Verification items for the finished model (mm, model axes). Round coordinates to 2 decimals unless told otherwise and drop trailing zeros. Order: outer loops, then holes, each group sorted by start corner. A loop starts at its lowest first (then second) coordinate and runs counter-clockwise, first axis right, second up. Notation, with made-up numbers: M 28,1 L 65,1 A20 ccw 65,35 Z; hole C 36,70 d5. An arc over 180 degrees is marked long. One line per item, written item: value. Start each with the question number.
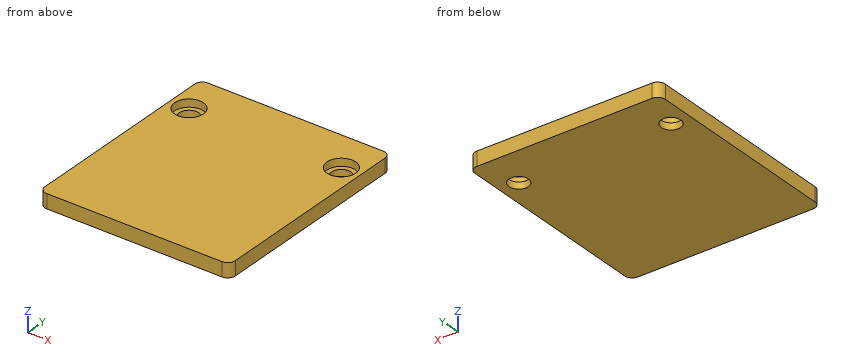
from build123d import *

# Parameters (mm, degrees)
SKETCH1_W                                        = 63.5
SKETCH1_H                                        = 71.4375
BOSS_EXTRUDE1_DEPTH                              = 4.7625
CBORE_FOR_1_4_SOCKET_HEAD_CAP_SCREW1_D           = 6.5278
CBORE_FOR_1_4_SOCKET_HEAD_CAP_SCREW1_CBORE_D     = 9.652
CBORE_FOR_1_4_SOCKET_HEAD_CAP_SCREW1_CBORE_DEPTH = 2.54
FILLET2_R                                        = 2.54


with BuildPart() as part:
    # Sketch1 → Boss-Extrude1 (new body)
    with BuildSketch(Plane.XY):
        with Locations((31.75, 35.71875)):
            Rectangle(SKETCH1_W, SKETCH1_H)
    extrude(amount=BOSS_EXTRUDE1_DEPTH)

    # CBORE for 1/4 Socket Head Cap Screw1 (through all)
    with Locations(Plane.XY.offset(4.7625)):
        with Locations((57.15, 57.9501), (6.35, 57.9501)):
            CounterBoreHole(CBORE_FOR_1_4_SOCKET_HEAD_CAP_SCREW1_D / 2, CBORE_FOR_1_4_SOCKET_HEAD_CAP_SCREW1_CBORE_D / 2, CBORE_FOR_1_4_SOCKET_HEAD_CAP_SCREW1_CBORE_DEPTH)

    # Fillet2
    fillet2_edges = [part.edges().sort_by_distance(p)[0] for p in [
        (0, 71.4375, 2.38125),
        (63.5, 71.4375, 2.38125),
        (63.5, 0, 2.38125),
        (0, 0, 2.38125),
    ]]
    fillet(fillet2_edges, radius=FILLET2_R)


solid = part.part
1. Section check B-B (z = 0.95). Record the cut outline in (x, y), and give its area (3 significant figures).
2. Scan lines: line 1 along Y through (x, z) = (6.35, 2.9); line 2 along X through (y, z) = (54, 2.7); line 3 along Y through (x, z) = (6.35, 1.05). Record each from-to range of solid material in increasing order.
3. Depth check by flat-ended pin: pin 1 (3 mm diameter, centred on x = 56, y = 55.5, fed in from +Z); pin 2 (7.5 mm diameter, centred on x = 57.15, y = 57.95, fed in from -Z); pin 3 (6 mm diameter, centred on x = 57.15, y = 57.95, fed in from -Z). Enter the tip coordinate at first touch or a pass-through.
4. Section check A-A (x = 57.15). Record the cut outline in (y, z), and give its area (3 significant figures).
Geometry check:
1. outline: M 0,2.54 A2.54 ccw 2.54,0 L 60.96,0 A2.54 ccw 63.5,2.54 L 63.5,68.9 A2.54 ccw 60.96,71.44 L 2.54,71.44 A2.54 ccw 0,68.9 Z; hole C 6.35,57.95 d6.53; hole C 57.15,57.95 d6.53
1. area: 4,460 mm²
2. line 1: y = 0 to 53.12, 62.78 to 71.44
2. line 2: x = 0 to 3.58, 9.12 to 54.38, 59.92 to 63.5
2. line 3: y = 0 to 54.69, 61.21 to 71.44
3. pin 1: stops at z = 2.22
3. pin 2: stops at z = 0
3. pin 3: passes through
4. outline: M 0,0 L 54.69,0 L 54.69,2.22 L 53.12,2.22 L 53.12,4.76 L 0,4.76 Z; M 61.21,0 L 71.44,0 L 71.44,4.76 L 62.78,4.76 L 62.78,2.22 L 61.21,2.22 Z
4. area: 301 mm²
